```python
from build123d import *

# Parameters (mm, degrees)
BOSS_EXTRUDE1_DEPTH                   = 139.7
F_1_8_0_125_DIAMETER_HOLE1_AT_2_COUNT = 2
F_1_8_0_125_DIAMETER_HOLE1_AT_2_PITCH = 66.3448
LPATTERN1_COUNT                       = 5
LPATTERN1_PITCH                       = 11.43


with BuildPart() as part:
    # Sketch1 → Boss-Extrude1 (new body)
    with BuildSketch(Plane.XY):
        with BuildLine():
            Line((-37.544302716, 7.712013675), (-44.529302716, 7.712013675))
            ThreePointArc((-44.529302716, 7.712013675), (-7.864402716, 44.376913675), (28.800497284, 7.712013675))
            Line((28.800497284, 7.712013675), (21.815497284, 7.712013675))
            ThreePointArc((21.815497284, 7.712013675), (-7.864402716, 37.391913675), (-37.544302716, 7.712013675))
        make_face()
    extrude(amount=BOSS_EXTRUDE1_DEPTH)

    # Sketch4 → 1/8 (0.125) Diameter Hole1 (revolve, cut)
    with BuildSketch(Plane(origin=(-41.036802716, 7.712013675, 76.2), x_dir=(0, 0, -1), z_dir=(1, 0, 0))):
        Polygon((0, 0), (0, 1.453866233), (1.5875, 0.5), (1.5875, 0), align=None)
    f_1_8_0_125_diameter_hole1 = revolve(axis=Axis((-41.036802716, 1.362013675, 76.2), (0, 1, 0)), mode=Mode.SUBTRACT)

    # 1/8 (0.125) Diameter Hole1 at 2: 1/8 (0.125) Diameter Hole1 ×2
    with Locations(*[(i * F_1_8_0_125_DIAMETER_HOLE1_AT_2_PITCH, 0, 0) for i in range(1, F_1_8_0_125_DIAMETER_HOLE1_AT_2_COUNT)]):
        add(f_1_8_0_125_diameter_hole1, mode=Mode.SUBTRACT)

    # LPattern1: 1/8 (0.125) Diameter Hole1 ×5
    with Locations(*[(0, 0, -i * LPATTERN1_PITCH) for i in range(1, LPATTERN1_COUNT)]):
        add(f_1_8_0_125_diameter_hole1, mode=Mode.SUBTRACT)

    # LPattern1 copy 1 sketch → LPattern1 copy 1 (revolve, cut)
    with BuildSketch(Plane(origin=(25.307997284, 7.712013675, 64.77), x_dir=(0, 0, -1), z_dir=(1, 0, 0))):
        Polygon((0, 0), (0, 1.453866233), (1.5875, 0.5), (1.5875, 0), align=None)
    revolve(axis=Axis((25.307997284, 1.362013675, 64.77), (0, 1, 0)), mode=Mode.SUBTRACT)

    # LPattern1 copy 2 sketch → LPattern1 copy 2 (revolve, cut)
    with BuildSketch(Plane(origin=(25.307997284, 7.712013675, 53.34), x_dir=(0, 0, -1), z_dir=(1, 0, 0))):
        Polygon((0, 0), (0, 1.453866233), (1.5875, 0.5), (1.5875, 0), align=None)
    revolve(axis=Axis((25.307997284, 1.362013675, 53.34), (0, 1, 0)), mode=Mode.SUBTRACT)

    # LPattern1 copy 3 sketch → LPattern1 copy 3 (revolve, cut)
    with BuildSketch(Plane(origin=(25.307997284, 7.712013675, 41.91), x_dir=(0, 0, -1), z_dir=(1, 0, 0))):
        Polygon((0, 0), (0, 1.453866233), (1.5875, 0.5), (1.5875, 0), align=None)
    revolve(axis=Axis((25.307997284, 1.362013675, 41.91), (0, 1, 0)), mode=Mode.SUBTRACT)

    # LPattern1 copy 4 sketch → LPattern1 copy 4 (revolve, cut)
    with BuildSketch(Plane(origin=(25.307997284, 7.712013675, 30.48), x_dir=(0, 0, -1), z_dir=(1, 0, 0))):
        Polygon((0, 0), (0, 1.453866233), (1.5875, 0.5), (1.5875, 0), align=None)
    revolve(axis=Axis((25.307997284, 1.362013675, 30.48), (0, 1, 0)), mode=Mode.SUBTRACT)


solid = part.part
```
The listing builds one solid part. Answer for the finished solid, in the listing's coordinates (mm). A direction names the side the tool comes from. Coordinates: 2 decimals unless noted, no trailing zeros. Write each loop counter-clockwise with the first axis right and the second up, starting at its lowest first coordinate (ties: lowest second). Pieces come first, ordered by that corner, then holes. Notation, with made-up numbers: (28.25, 26) - (64.25, 26) arc R29 cw to (64.25, 46) - close; hole circle Ø2 at (2, 17). An arc over 180 degrees is marked (long way). One line per item, written item: value.
1) Find section B-B (x = -7). Give the vertices of the cut face in (y, z).
Geometry check:
outline: (37.38, 0) - (44.37, 0) - (44.37, 139.7) - (37.38, 139.7) - close
2) Find section A-A (z = 87.5). Give the vertices of the cut face in (x, y).
Geometry check:
outline: (-44.53, 7.71) - (-37.54, 7.71) arc R29.68 cw to (21.82, 7.71) - (28.8, 7.71) arc R36.66 ccw to start
3) A tool of negligible diameter and unlimited length cuts with its end or side. For faces 1 (the cylindrical face through (26.716, 7.959, 64.037)), 2 (the flat face through (-2, 37, 0)), from which of +Z, -Z, +X, -X, +Y, -Y can it reach the whole face along a straight path? Write none if from no direction.
Geometry check:
face 1: -Y
face 2: -Z, +X, -X, +Y, -Y
4) Consider line 1 along X through (y, z) = (8.1, 76.2); line 2 along X through (y, z) = (16.5, 59); line 3 along X through (y, z) = (8, 30). Determine where each line is inside the solid, lowest interval first. Write a range as from..to.
Geometry check:
line 1: x = -44.53..-42.62, -39.45..-37.54, 21.81..23.72, 26.9..28.8
line 2: x = -43.46..-36.21, 20.48..27.73
line 3: x = -44.53..-42.55, -39.52..-37.54, 21.81..23.79, 26.82..28.8
5) For a pull along X with two mould halves and no side action, classify faces 3 (the flat face through (-2, 37, 139.7)), 4 (the conical face through (-40.87, 9, 42.13)) as pulls with the +X half, pulls with the -X half, needs draft (parallel to the pull), parting line crosses it, or undercut.
Geometry check:
face 3: needs draft
face 4: undercut
6) Each of these flat-tipped pins is pushed along its axis until it touches: pin 1 Ø3 at (x, z) = (25.31, 41.91) entering from +Y; pin 2 Ø4 at (y, z) = (26.5, 58.5) entering from -X; pin 3 Ø2.5 at (x, z) = (25.31, 76.2) entering from -Y. Where does it stop, or does it pass through?
Geometry check:
pin 1: stops at y = 26.18
pin 2: stops at x = -40.46
pin 3: stops at y = 8.41
